```python
from build123d import *

# Parameters (mm, degrees)
BASE_EXTRUDE_DEPTH  = 12.7
BOSS_EXTRUDE2_START = -11.060769
SKETCH2_W           = 12.7
SKETCH2_H           = 16.891
BOSS_EXTRUDE2_DEPTH = 11.060769
SKETCH3_W           = 12.7
SKETCH3_H           = 16.891
BOSS_EXTRUDE3_DEPTH = 25.4
FILLET1_R           = 17.78


with BuildPart() as part:
    # Sketch1 → Base-Extrude (new body)
    with BuildSketch(Plane.XY):
        with BuildLine():
            Line((-43.18, 0), (-17.78, 0))
            ThreePointArc((-17.78, 0), (0, 17.78), (17.78, 0))
            Line((17.78, 0), (43.18, 0))
            ThreePointArc((43.18, 0), (0, 43.18), (-43.18, 0))
        make_face()
    extrude(amount=BASE_EXTRUDE_DEPTH)

    # Sketch2 → Boss-Extrude2 (add)
    with BuildSketch(Plane(origin=(50.8, 0, 0), x_dir=(0, 0, -1), z_dir=(1, 0, 0)).offset(BOSS_EXTRUDE2_START)):
        with Locations((-6.35, 8.4455)):
            Rectangle(SKETCH2_W, SKETCH2_H)
    extrude(amount=BOSS_EXTRUDE2_DEPTH)

    # Sketch3 → Boss-Extrude3 (add)
    with BuildSketch(Plane(origin=(50.8, 0, 0), x_dir=(0, 0, -1), z_dir=(1, 0, 0))):
        with Locations((-6.35, 8.4455)):
            Rectangle(SKETCH3_W, SKETCH3_H)
    extrude(amount=BOSS_EXTRUDE3_DEPTH)

    # Fillet1
    fillet1_edges = [part.edges().sort_by_distance(p)[0] for p in [
        (39.739231, 16.891, 6.35),
    ]]
    fillet(fillet1_edges, radius=FILLET1_R)


solid = part.part
```
Input: part model. Units: mm. Frame: model coordinates. A direction names the side the tool comes from. Give positions to 0.01 mm unless a question says otherwise; leave off trailing zeros. Order: outer loops, then holes, each group sorted by start corner. A loop starts at its lowest first (then second) coordinate and runs counter-clockwise, first axis right, second up. Notation, with made-up numbers: M 18.25,-17 L 25.25,-17 A21 ccw 25.25,5 Z; hole C -29,52 d7. An arc over 180 degrees is marked long. Return JSON: item names as keys, results as strings.
1) Mould query, pull axis X, two halves, no side actions, for faces 3 (the face through (-0.391, 17.776, 6.261)), 4 (the face through (76.2, 9, 6)), 5 (the face through (-12.13, 41.44, 6.26)). Classes: released by +X, released by -X, zero draft, split by the parting line, or undercut.
Taken from the geometry:
{"face 3": "undercut", "face 4": "released by +X", "face 5": "split by the parting line"}
2) Section query C-C on x = 0. Output: boundary loops of the cut face in (y, z), and give its area (3 significant figures).
Taken from the geometry:
{"outline": "M 17.78,0 L 43.18,0 L 43.18,12.7 L 17.78,12.7 Z", "area": "323 mm2"}
3) Section query A-A on z = 5. Output: boundary loops of the cut face in (x, y).
Taken from the geometry:
{"outline": "M -43.18,0 L -17.78,0 A17.78 cw 17.78,0 L 76.2,0 L 76.2,16.89 L 50.14,16.89 A17.78 cw 35.52,24.56 A43.18 ccw Z"}
4) Section query B-B on x = 52. Output: boundary loops of the cut face in (y, z).
Taken from the geometry:
{"outline": "M 0,0 L 16.89,0 L 16.89,12.7 L 0,12.7 Z"}
5) Line query: L1, parallel to X at y = 5, z = 2.5; L2, parallel to X at y = 10, z = 3.5; L3, parallel to Y at x = 55, z = 7. Output: solid intervals per line, ascending. Write a range as [from, to].
Taken from the geometry:
{"L1": "x = [-42.89, -17.06], [17.06, 76.2]", "L2": "x = [-42.01, -14.7], [14.7, 76.2]", "L3": "y = [0, 16.89]"}
6) Contact query for flat-ended pins moving along their axis: pin 1 (1.5 mm diameter, centred on y = 35, z = 9.5, fed in from -X); pin 2 (1 mm diameter, centred on y = 5, z = 7.5, fed in from -X); pin 3 (4 mm diameter, centred on x = -0.5, z = 10, fed in from +Y). Output: stop coordinate, or through.
Taken from the geometry:
{"pin 1": "stops at x = -26.3", "pin 2": "stops at x = -42.94", "pin 3": "stops at y = 43.18"}
7) Access query for faces 1 (the face through (63, 16.891, 6)), 2 (the face through (16, 16, 0)). Directions: +Z, -Z, +X, -X, +Y, -Y. A direction counts if a zero-diameter tool reaches every point of the face in a straight line with its end or side. Return the directions, or none.
Taken from the geometry:
{"face 1": "+Z, -Z, +X, +Y", "face 2": "-Z, +X, -X, +Y, -Y"}
